Geometry check sheet. Reference: the model listing, model coordinates, mm. A direction names the side the tool comes from. Give positions to 0.01 mm unless a question says otherwise; leave off trailing zeros. Loops run counter-clockwise (first coordinate to the right, second up) from the corner with the lowest first, then second, coordinate; pieces in that order, holes last.
1. Cross-section at B-B, the plane y = 2.5. State how many separate pieces and enclosed holes the cut face has, plus the area to 3 significant figures.
2. Cross-section at D-D, the plane z = 6. Record the cut outline in (x, y), plus the area to 3 significant figures.
3. Cross-section at A-A, the plane x = -84. Record the cut outline in (y, z).
4. Go/stop test with flat-tipped pins: pin 1 Ø3 at (x, y) = (-197.5, 4.5) entering from +Z; pin 2 Ø3 at (y, z) = (2, -13.5) entering from +X; pin 3 Ø1 at (x, y) = (-150.5, 2.5) entering from +Z; pin 4 Ø1 at (y, z) = (2, -9.5) entering from -X. Record where each tip stops, or that it passes through.
5. Cross-section at C-C, the plane x = 188. Record the cut outline in (y, z), plus the area to 3 significant figures.
6. Tool access check on faces 4 (the flat face through (152.449, 2.958, 54.316)), 5 (the cylindrical face through (185.77, 2.96, 63.5)). Record the directions out of +Z, -Z, +X, -X, +Y, -Y that give a thin tool (end or side, any length) a straight path to the whole face; none if there is none.
7. Release check for a two-part mould opening along X. For faces 1 (the flat face through (-175.636, 2.958, 12.572)), 2 (the flat face through (3, 6, 6)), 3 (the flat face through (-152.449, 2.958, 54.316)) record: +X half, -X half, draft (parallel to the pull), parting line (faces both ways), or undercut.
8. Material ranges on L1, parallel to X at y = 4.45, z = -24; L2, parallel to X at y = 2.7, z = 67; L3, parallel to X at y = 5.2, z = -13, recorded low to high.
from build123d import *

# Parameters (mm, degrees)
ESQUISSE1_R             = 4.15
ESQUISSE1_R_2           = 2
ESQUISSE1_R_3           = 2.65
BOSS_EXTRU_1_DEPTH      = 6
CHANFREIN1_SIZE         = 5
ESQUISSE3_R             = 1.8
ESQUISSE3_W             = 7
ESQUISSE3_H             = 9.3
ENL_V_MAT_EXTRU_1_DEPTH = 6


with BuildPart() as part:
    # Esquisse1 → Boss.-Extru.1 (new body)
    with BuildSketch(Plane(origin=(0, 0, 0), x_dir=(1, 0, 0), z_dir=(0, 1, 0))):
        Polygon((-150, 0), (-202, -25.5), (-202, -30.5), (-191.5, -30.5), (-191.5, -37.5), (-202, -37.5), (-202, -86), (-162, -86), (-162, -59), (-142.62745098, -49.5), (0, -49.5), (0, -37.5), (-150, -37.5), (-150, -30.5), (0, -30.5), (0, 0), (0, 44), (-150, 44), align=None)
        with Locations((-188, -67)):
            Circle(ESQUISSE1_R, mode=Mode.SUBTRACT)
        with Locations((-171, -34)):
            Circle(ESQUISSE1_R_2, mode=Mode.SUBTRACT)
        with Locations((-170, -67)):
            Circle(ESQUISSE1_R_3, mode=Mode.SUBTRACT)
        with Locations((-143.5, -18)):
            Circle(ESQUISSE1_R_2, mode=Mode.SUBTRACT)
    extrude(amount=BOSS_EXTRU_1_DEPTH)

    # Chanfrein1
    chanfrein1_edges = [part.edges().sort_by_distance(p)[0] for p in [
        (-162, 3, 86),
        (-202, 3, 86),
    ]]
    chamfer(chanfrein1_edges, length=CHANFREIN1_SIZE)

    # Esquisse3 → Enlèv. mat.-Extru.1 (cut)
    with BuildSketch(Plane(origin=(0, 6, 0), x_dir=(1, 0, 0), z_dir=(0, 1, 0))):
        with Locations((-143.5, 24)):
            Circle(ESQUISSE3_R)
        with Locations((-143.5, 35.65)):
            Rectangle(ESQUISSE3_W, ESQUISSE3_H)
        with Locations((-143.5, 12.35)):
            Rectangle(ESQUISSE3_W, ESQUISSE3_H)
    extrude(amount=-ENL_V_MAT_EXTRU_1_DEPTH, mode=Mode.SUBTRACT)

    # Symétrie1: part across plane


with BuildPart() as part_1:
    add(part.part)
    add(part.part.mirror(Plane(origin=(0, 6, 30.5), x_dir=(0, 0, 1), z_dir=(-1, 0, 0))))


solid = part_1.part
Result:
1. separate pieces: 1
1. enclosed holes: 15
1. area: 32,200 mm2
2. outline: (-162.24, 0) - (162.24, 0) - (162.24, 6) - (-162.24, 6) - close
2. area: 1,950 mm2
3. outline: (0, -44) - (6, -44) - (6, 30.5) - (0, 30.5) - close; (0, 37.5) - (6, 37.5) - (6, 49.5) - (0, 49.5) - close
4. pin 1: stops at z = 86
4. pin 2: stops at x = 150
4. pin 3: stops at z = 53.61
4. pin 4: stops at x = -150
5. outline: (0, 18.63) - (6, 18.63) - (6, 62.85) - (0, 62.85) - close; (0, 71.15) - (6, 71.15) - (6, 86) - (0, 86) - close
5. area: 354 mm2
6. face 4: +Z, +Y, -Y
6. face 5: +Y, -Y
7. face 1: -X half
7. face 2: draft
7. face 3: undercut
8. L1: x = -150 to -145.3, -141.7 to 141.7, 145.3 to 150
8. L2: x = -202 to -192.15, -183.85 to -172.65, -167.35 to -162, 162 to 167.35, 172.65 to 183.85, 192.15 to 202
8. L3: x = -150 to -147, -140 to 140, 147 to 150
